```python
from build123d import *

# Parameters (mm, degrees)
SKETCH_1_W          = 80
SKETCH_1_H          = 60
EXTRUDE_1_DEPTH     = 20
SKETCH_2_W          = 61
SKETCH_2_H          = 60
CUT_EXTRUDE_1_DEPTH = 14
SKETCH_3_R          = 19.05
CUT_EXTRUDE_2_DEPTH = 54.851648071
M4X0_7_1_D          = 3.3


with BuildPart() as part:
    # 草圖1 → 填料-伸長1 (new body)
    with BuildSketch(Plane.XY):
        Rectangle(SKETCH_1_W, SKETCH_1_H)
    extrude(amount=EXTRUDE_1_DEPTH)

    # 草圖2 → 除料-伸長1 (cut)
    with BuildSketch(Plane.XY.offset(20)):
        Rectangle(SKETCH_2_W, SKETCH_2_H)
    extrude(amount=-CUT_EXTRUDE_1_DEPTH, mode=Mode.SUBTRACT)

    # 草圖3 → 除料-伸長2 (cut, through all)
    with BuildSketch(Plane(origin=(0, 0, 0), x_dir=(-1, 0, 0), z_dir=(0, 0, -1))):
        Circle(SKETCH_3_R)
    extrude(amount=-CUT_EXTRUDE_2_DEPTH, mode=Mode.SUBTRACT)

    # M4x0.7 螺紋孔1 (through all)
    with Locations(Plane(origin=(0, 0, 0), x_dir=(-1, 0, 0), z_dir=(0, 0, -1))):
        with Locations((23.57, 23.57), (-23.57, -23.57), (-23.57, 23.57), (23.57, -23.57)):
            Hole(M4X0_7_1_D / 2)


solid = part.part
```
The listing builds one solid part. Answer for the finished solid, in the listing's coordinates (mm). A direction names the side the tool comes from. Give positions to 0.01 mm unless a question says otherwise; leave off trailing zeros. Order: outer loops, then holes, each group sorted by start corner. A loop starts at its lowest first (then second) coordinate and runs counter-clockwise, first axis right, second up. Notation, with made-up numbers: (46.5, 1) - (91.5, 1) arc R17 cw to (91.5, 13) - close; hole circle Ø5 at (86, -1). An arc over 180 degrees is marked (long way). Answer in a Markdown table with one row per item. Add a question column.
Q1. The part is cut by section C-C (x = 0). Determine the outline of the cut face in (y, z), then the cut area to 3 significant figures.
Q2. The part is cut by section D-D (y = 23.57). Determine the outline of the cut face in (x, z), then the cut area to 3 significant figures.
Q3. Find the intervals of material crossed by line 1 along Y through (x, z) = (23.57, 3.2); line 2 along X through (y, z) = (-22, 14.25); line 3 along Y through (x, z) = (0, 1.6), in increasing order. Write a range as [from, to].
Q4. The part is cut by section B-B (z = 12). Determine the outline of the cut face in (x, y).
Q5. Given P1, Ø4, axis at x = 23.57, y = -23.57, coming from the -Z side; P2, Ø10, axis at x = -7, y = 16, coming from the +Z side, each flat-ended and moving along its own axis, determine where each tip first touches the part or whether it passes through.
Q6. For a pull along X with two mould halves and no side action, classify faces 1 (the flat face through (40, 0, 10)), 2 (the flat face through (-18.3, -6.2, 0)), 3 (the cylindrical face through (15.12, -11.59, 2.96)), 4 (the flat face through (-30.5, 0, 13)) as released by +X, released by -X, zero draft, split by the parting line, or undercut.
Q7. The part is cut by section A-A (x = -23.57). Determine the outline of the cut face in (y, z), then the cut area to 3 significant figures.
Q8. Which of the six approach directions +Z, -Z, +X, -X, +Y, -Y give full straight-line access (tool end or side, diameter ignored) to faces 5 (the flat face through (-1, -30, 5)), 6 (the flat face through (-14, 14, 6))?
Determined:
| question | item | result |
|---|---|---|
| 1 | outline | (-30, 0) - (-19.05, 0) - (-19.05, 6) - (-30, 6) - close; (19.05, 0) - (30, 0) - (30, 6) - (19.05, 6) - close |
| 1 | area | 131 mm² |
| 2 | outline | (-40, 0) - (-25.22, 0) - (-25.22, 6) - (-30.5, 6) - (-30.5, 20) - (-40, 20) - close; (-21.92, 0) - (21.92, 0) - (21.92, 6) - (-21.92, 6) - close; (25.22, 0) - (40, 0) - (40, 20) - (30.5, 20) - (30.5, 6) - (25.22, 6) - close |
| 2 | area | 706 mm² |
| 3 | line 1 | y = [-30, -25.22], [-21.92, 21.92], [25.22, 30] |
| 3 | line 2 | x = [-40, -30.5], [30.5, 40] |
| 3 | line 3 | y = [-30, -19.05], [19.05, 30] |
| 4 | outline | (-40, -30) - (-30.5, -30) - (-30.5, 30) - (-40, 30) - close; (30.5, -30) - (40, -30) - (40, 30) - (30.5, 30) - close |
| 5 | P1 | stops at z = 0 |
| 5 | P2 | stops at z = 6 |
| 6 | face 1 | released by +X |
| 6 | face 2 | zero draft |
| 6 | face 3 | undercut |
| 6 | face 4 | undercut |
| 7 | outline | (-30, 0) - (-25.22, 0) - (-25.22, 6) - (-30, 6) - close; (-21.92, 0) - (21.92, 0) - (21.92, 6) - (-21.92, 6) - close; (25.22, 0) - (30, 0) - (30, 6) - (25.22, 6) - close |
| 7 | area | 320 mm² |
| 8 | face 5 | +Z, -Z, +X, -X, -Y |
| 8 | face 6 | +Z, +Y, -Y |
